The model under review builds one solid part; all positions refer to its coordinate system, in mm. Face numbers are marked on the shaded views. A direction names the side the tool comes from. Coordinates: 2 decimals unless noted, no trailing zeros. Loops run counter-clockwise (first coordinate to the right, second up) from the corner with the lowest first, then second, coordinate; pieces in that order, holes last. Notation, with made-up numbers: M 48.5,19 L 62.5,19 A11 cw 62.5,39 Z; hole C 17.5,48.5 d9. An arc over 180 degrees is marked long. Use CSV: the item, a comma, the result in double quotes. Start each with the question number.
1. Draft analysis for pull direction Y (two halves, no side actions). For the marked faces 1, 2 and 3, state which applies: +Y half, -Y half, draft (parallel to the pull), parting line (faces both ways), or undercut.
2. Add section A-A, the plane y = 0. Write out the cut boundary in (x, z).
3. Add section C-C, the plane z = 2. Write out the cut boundary in (x, y).
4. For L1, parallel to X at y = -0.25, z = 7.25; L2, parallel to Y at x = 0, z = 7; L3, parallel to Z at x = 1, y = -9.5, list the stretches that pass through material, from the lowest coordinate up.
5. Add section D-D, the plane y = 7. Write out the cut boundary in (x, z), then the cut area to 3 significant figures.
6. Clearance check with flat-ended pins moving along their axes: P1, Ø8, axis at y = 3.5, z = 8.5, coming from the +X side; P2, Ø1.5, axis at y = -7.5, z = 3.5, coming from the +X side; P3, Ø6, axis at x = -1, z = 11.5, coming from the -Y side. State where each tip first meets the part, or that it passes through.
7. Tool access review of the marked faces 4 and 5: name each direction out of +Z, -Z, +X, -X, +Y, -Y from which nothing blocks a thin tool from reaching the whole face with its end or side.
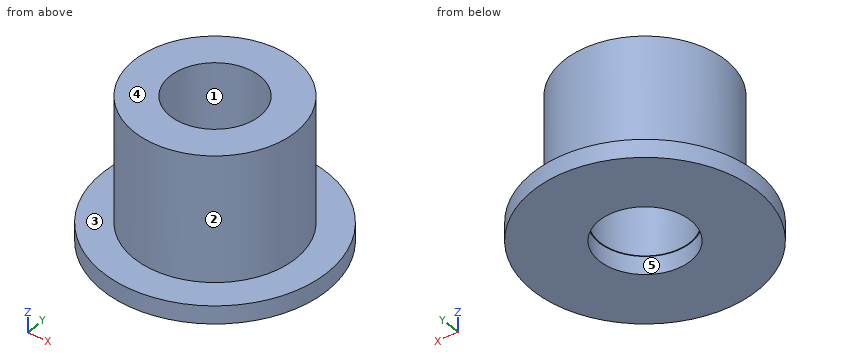
from build123d import *

# Parameters (mm, degrees)
F0_R     = 9
F0_R_2   = 5
F1_DEPTH = 14
F2_R     = 12.5
F2_R_2   = 5.083176
F3_DEPTH = 2


with BuildPart() as f1:
    # F0 (on Top) → F1 (new body)
    with BuildSketch(Plane.XY):
        Circle(F0_R)
        Circle(F0_R_2, mode=Mode.SUBTRACT)
    extrude(amount=F1_DEPTH)

    # F2 (on Top) → F3 (join)
    with BuildSketch(Plane.XY):
        Circle(F2_R)
        Circle(F2_R_2, mode=Mode.SUBTRACT)
    extrude(amount=-F3_DEPTH)


solid = f1.part
Computed:
1,face 1,"undercut"
1,face 2,"parting line"
1,face 3,"draft"
2,outline,"M -12.5,-2 L -5.08,-2 L -5.08,0 L -5,0 L -5,14 L -9,14 L -9,0 L -12.5,0 Z; M 5,0 L 5.08,0 L 5.08,-2 L 12.5,-2 L 12.5,0 L 9,0 L 9,14 L 5,14 Z"
3,outline,"C 0,0 d18; hole C 0,0 d10"
4,L1,"x = -9 to -4.99, 4.99 to 9"
4,L2,"y = -9 to -5, 5 to 9"
4,L3,"z = -2 to 0"
5,outline,"M -10.36,-2 L 10.36,-2 L 10.36,0 L 5.66,0 L 5.66,14 L -5.66,14 L -5.66,0 L -10.36,0 Z"
5,area,"200 mm^2"
6,P1,"stops at x = 9"
6,P2,"stops at x = 5.95"
6,P3,"stops at y = -9"
7,face 4,"+Z, +X, -X, +Y, -Y"
7,face 5,"-Z"
